For this review, use the dimensioned drawing (mm, ordinates from the lowest corner) and the shaded views. Coordinates: 2 decimals unless noted, no trailing zeros. Write each loop counter-clockwise with the first axis right and the second up, starting at its lowest first coordinate (ties: lowest second). Pieces come first, ordered by that corner, then holes. Notation, with made-up numbers: M 72.25,37 L 123.25,37 A13 ccw 123.25,42 Z; hole C -25.75,26.5 d9. An arc over 180 degrees is marked long. One line per question, with ' | ' between items.
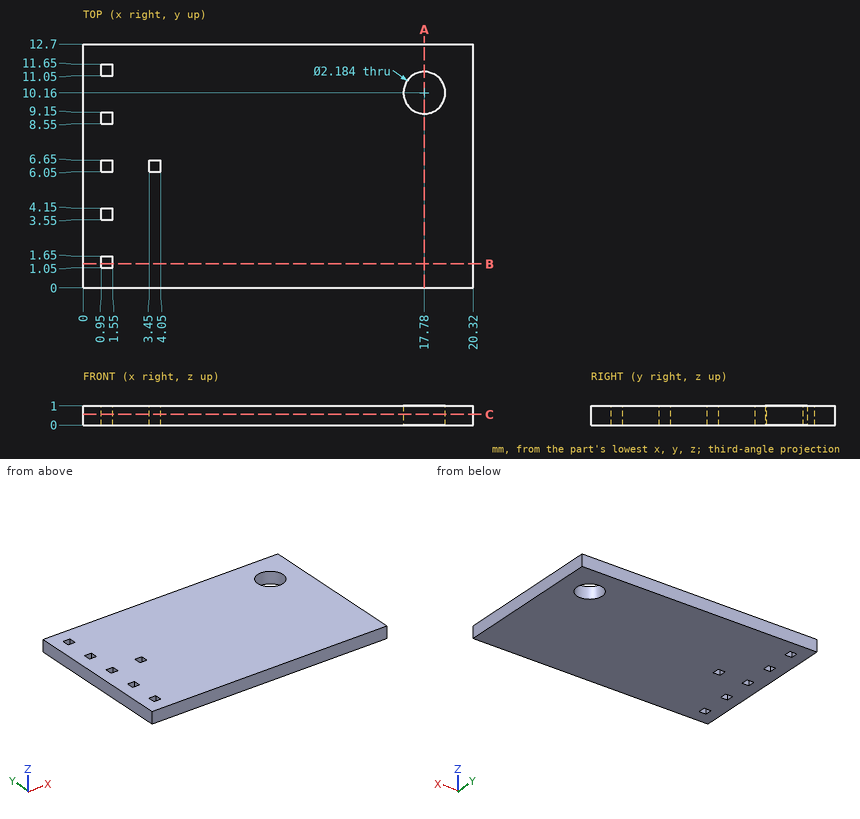
1. Take a section at B-B (y = 1.25). Write out the cut boundary in (x, z).
Answer sheet:
outline: M 0,0 L 0.95,0 L 0.95,1 L 0,1 Z; M 1.55,0 L 20.32,0 L 20.32,1 L 1.55,1 Z
2. Take a section at C-C (z = 0.55). Count the separate pieces of the cut face and the enclosed holes in it, then the cut area to 3 significant figures.
Answer sheet:
separate pieces: 1 | enclosed holes: 7 | area: 252 mm^2
3. Take a section at A-A (x = 17.78). Write out the cut boundary in (y, z), then the cut area to 3 significant figures.
Answer sheet:
outline: M 0,0 L 9.07,0 L 9.07,1 L 0,1 Z; M 11.25,0 L 12.7,0 L 12.7,1 L 11.25,1 Z | area: 10.5 mm^2
4. To check wall thickness, follow line 1 along Y through (x, z) = (1, 0.5); line 2 along Y through (x, z) = (4, 0.35); line 3 along Y through (x, z) = (17.78, 0.45). State the ranges of each line that lie inside material, in increasing order. Write a range as [from, to].
Answer sheet:
line 1: [0, 1.05], [1.65, 3.55], [4.15, 6.05], [6.65, 8.55], [9.15, 11.05], [11.65, 12.7] | line 2: [0, 6.05], [6.65, 12.7] | line 3: [0, 9.07], [11.25, 12.7]
